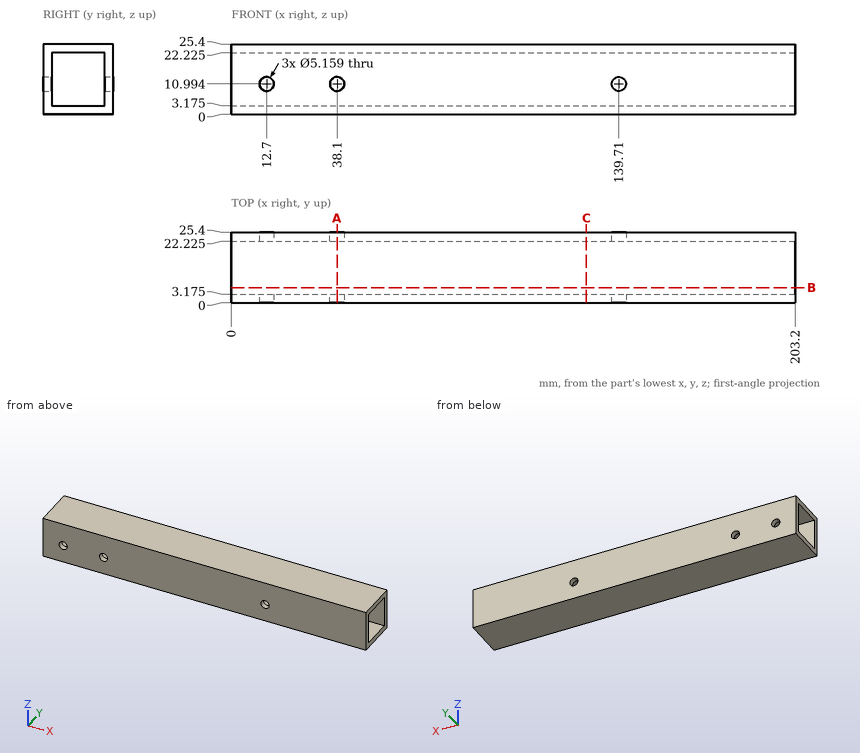
Geometry check sheet. Reference: drawing and pictorial views, mm from the part's lowest x, y, z. Give positions to 0.01 mm unless a question says otherwise; leave off trailing zeros. Write each loop counter-clockwise with the first axis right and the second up, starting at its lowest first coordinate (ties: lowest second). Pieces come first, ordered by that corner, then holes. Notation, with made-up numbers: (-10, 24.5) - (27, 24.5) arc R10 cw to (27, 36.5) - close; hole circle Ø2 at (-8, 79). An arc over 180 degrees is marked (long way). Use a Markdown table: item, result.
Q1. Section check A-A, the plane x = 38.1. Enter the section's corners in (y, z) (1 decimal).
Computed:
| item | result |
|---|---|
| outline | (0, 0) - (25.4, 0) - (25.4, 8.4) - (22.2, 8.4) - (22.2, 3.2) - (3.2, 3.2) - (3.2, 8.4) - (0, 8.4) - close; (0, 13.6) - (3.2, 13.6) - (3.2, 22.2) - (22.2, 22.2) - (22.2, 13.6) - (25.4, 13.6) - (25.4, 25.4) - (0, 25.4) - close |
Q2. Section check C-C, the plane x = 128. Enter the section's corners in (y, z) (1 decimal).
Computed:
| item | result |
|---|---|
| outline | (0, 0) - (25.4, 0) - (25.4, 25.4) - (0, 25.4) - close; hole (3.2, 3.2) - (22.2, 3.2) - (22.2, 22.2) - (3.2, 22.2) - close |
Q3. Thickness scan on L1, parallel to Z at x = 191.5, y = 16.75 (1 decimal); L2, parallel to Z at x = 12.7, y = 22.9. Record the ranges inside material, lowest first. Write a range as [from, to].
Computed:
| item | result |
|---|---|
| L1 | z = [0, 3.2], [22.2, 25.4] |
| L2 | z = [0, 8.41], [13.57, 25.4] |
Q4. Section check B-B, the plane y = 5.5. Enter the section's corners in (x, z) (1 decimal).
Computed:
| item | result |
|---|---|
| outline | (0, 0) - (203.2, 0) - (203.2, 3.2) - (0, 3.2) - close; (0, 22.2) - (203.2, 22.2) - (203.2, 25.4) - (0, 25.4) - close |
